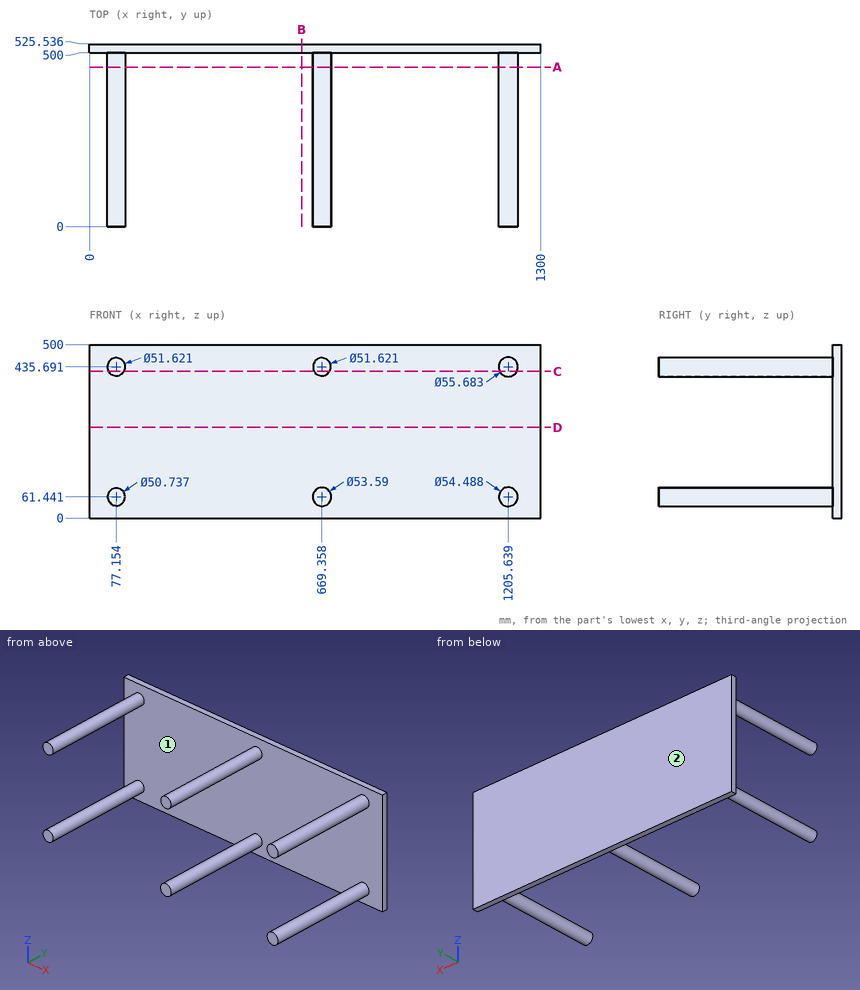
Source: three-view drawing plus pictorial views. Frame: mm from the lowest corner of the part. Give positions to 0.01 mm unless a question says otherwise; leave off trailing zeros. Write each loop counter-clockwise with the first axis right and the second up, starting at its lowest first coordinate (ties: lowest second). Pieces come first, ordered by that corner, then holes. Notation, with made-up numbers: (17.5, -16.5) - (33.5, -16.5) arc R15 cw to (33.5, -6.5) - close; hole circle Ø2 at (10, 40). An arc over 180 degrees is marked (long way). Write item = value, one per line. Start each with the question number.
1. Ray query, L1, parallel to X at y = 477, z = 435 (1 decimal); L2, parallel to X at y = 30, z = 428.5 (1 decimal); L3, parallel to Y at x = 1144, z = 171.5 (1 decimal). Return the intervals inside material, ascending.
2. First-contact query: pin 1 Ø6 at (x, z) = (1059, 440.5) entering from -Y. Flat tip, straight axial feed; report the tip coordinate or a pass-through.
3. Section query B-B, the plane x = 611. Output: boundary loops of the cut face in (y, z) (1 decimal).
4. Section query C-C, the plane z = 423. Output: boundary loops of the cut face in (x, y) (1 decimal), then the cut area to 3 significant figures.
5. Section query D-D, the plane z = 261.5. Output: boundary loops of the cut face in (x, y) (1 decimal), then the cut area to 3 significant figures.
6. Section query A-A, the plane y = 459. Output: boundary loops of the cut face in (x, z) (1 decimal).
7. Mould query, pull axis X, two halves, no side actions, for the marked faces 1 and 2. Classes: released by +X, released by -X, zero draft, split by the parting line, or undercut.
Check sheet entries:
q1.L1 = 51.4 to 103, 643.6 to 695.2, 1177.8 to 1233.5
q1.L2 = 52.4 to 101.9, 644.6 to 694.1, 1178.7 to 1232.5
q1.L3 = 500 to 525.5
q2.pin_1 = 500
q3.outline = (500, 0) - (525.5, 0) - (525.5, 500) - (500, 500) - close
q4.outline = (0, 500) - (54.7, 500) - (54.7, 0) - (99.6, 0) - (99.6, 500) - (646.9, 500) - (646.9, 0) - (691.8, 0) - (691.8, 500) - (1180.9, 500) - (1180.9, 0) - (1230.4, 0) - (1230.4, 500) - (1300, 500) - (1300, 525.5) - (0, 525.5) - close
q4.area = 103,000 mm2
q5.outline = (0, 500) - (1300, 500) - (1300, 525.5) - (0, 525.5) - close
q5.area = 33,200 mm2
q6.outline = circle Ø51.6 at (77.2, 435.7); circle Ø50.7 at (77.2, 61.4); circle Ø53.6 at (669.4, 61.4); circle Ø51.6 at (669.4, 435.7); circle Ø55.7 at (1205.6, 435.7); circle Ø54.5 at (1205.6, 61.4)
q7.face_1 = undercut
q7.face_2 = zero draft
